Could you check a few things on this model? Use its own coordinates, in mm. A direction names the side the tool comes from. Give positions to 0.01 mm unless a question says otherwise; leave off trailing zeros. Loops run counter-clockwise (first coordinate to the right, second up) from the corner with the lowest first, then second, coordinate; pieces in that order, holes last. Notation, with made-up numbers: M 58,-1 L 81,-1 A14 ccw 81,3 Z; hole C 5,49 d8. An arc over 180 degrees is marked long. Use CSV: the item, a comma, the result in double quotes.
```python
from build123d import *

# Parameters (mm, degrees)
F0_R     = 15
F1_DEPTH = 150
F2_W     = 20
F2_H     = 20
F3_DEPTH = 25
F4_DEPTH = 25


with BuildPart() as f1:
    # F0 (on Top) → F1 (new body)
    with BuildSketch(Plane.XY):
        Circle(F0_R)
    extrude(amount=F1_DEPTH)

    # F2 (on Right) → F3 (cut)
    with BuildSketch(Plane.YZ):
        with Locations((1.143422, 125)):
            Rectangle(F2_W, F2_H)
    extrude(amount=-F3_DEPTH, mode=Mode.SUBTRACT)

    # F2 (on Right) → F4 (cut)
    with BuildSketch(Plane.YZ):
        with Locations((1.143422, 125)):
            Rectangle(F2_W, F2_H)
    extrude(amount=F4_DEPTH, mode=Mode.SUBTRACT)


solid = f1.part
```
1. I want a section at A-A, the plane y = 6. List the corners of the cut face in (x, z) for me.
Outcome:
outline,"M -13.75,0 L 13.75,0 L 13.75,115 L -13.75,115 Z; M -13.75,135 L 13.75,135 L 13.75,150 L -13.75,150 Z"
2. I want a section at D-D, the plane y = 0. List the corners of the cut face in (x, z) for me.
Outcome:
outline,"M -15,0 L 15,0 L 15,115 L -15,115 Z; M -15,135 L 15,135 L 15,150 L -15,150 Z"
3. I want a section at B-B, the plane x = 0. List the corners of the cut face in (y, z) for me, then the cut area to 3 significant figures.
Outcome:
outline,"M -15,0 L 15,0 L 15,150 L -15,150 Z; hole M -8.86,115 L 11.14,115 L 11.14,135 L -8.86,135 Z"
area,"4,100 mm2"
4. If we mould it in two halves opening along Z, with no side actions, what happens to faces 1 (the face through (0, 0, 0)), 2 (the face through (0, 1, 135)), 3 (the face through (0, 0, 150))? For each: +Z half, -Z half, draft (parallel to the pull), parting line (faces both ways), or undercut.
Outcome:
face 1,"-Z half"
face 2,"undercut"
face 3,"+Z half"
5. Please list where these lines run through material, in increasing order: line 1 (Z direction, x = -13, y = -2.5); line 2 (Y direction, x = 0.25, z = 79); line 3 (Y direction, x = 3, z = 128.5).
Outcome:
line 1,"0 to 115, 135 to 150"
line 2,"-15 to 15"
line 3,"-14.7 to -8.86, 11.14 to 14.7"
6. I want a section at C-C, the plane z = 84. List the corners of the cut face in (x, y) for me.
Outcome:
outline,"C 0,0 d30"
7. Which directions (+Z, -Z, +X, -X, +Y, -Y) give clear straight access to the entire face, cutting with the end or side of a thin tool? Please do faces 4 (the face through (0, -8.857, 125)), 5 (the face through (-3.252, -14.643, 73.95)).
Outcome:
face 4,"+X, -X"
face 5,"+Z, -Z"
8. I'm going to push flat-ended pins straight in: pin 1 Ø6 at (x, z) = (-4.5, 121) entering from -Y; pin 2 Ø5 at (y, z) = (10.5, 21.5) entering from -X; pin 3 Ø10 at (x, z) = (-5.5, 128.5) entering from +Y. Where does each tip first touch, or does it pass through?
Outcome:
pin 1,"y = -14.92"
pin 2,"x = -12.69"
pin 3,"y = 14.99"
